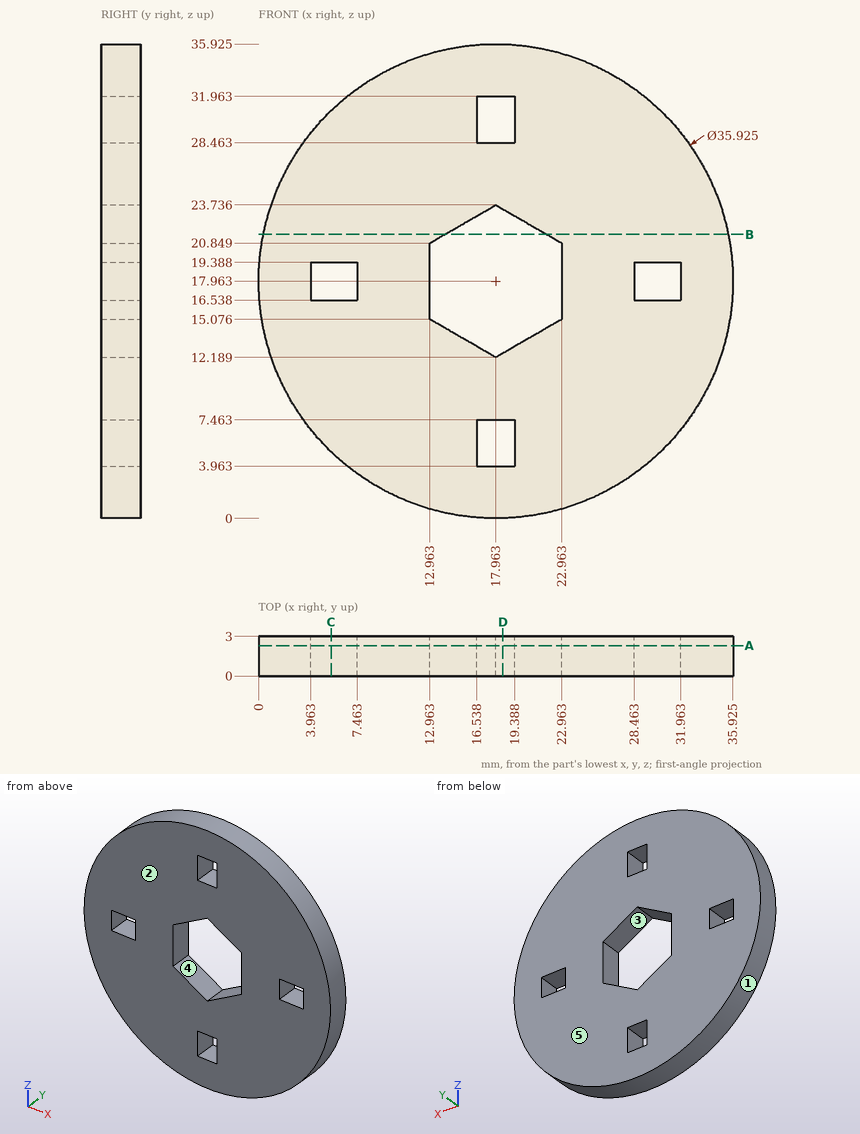
Answer from the drawing. Dimensions are ordinates in mm from the lowest x, y and z of the part. A direction names the side the tool comes from. Give positions to 0.01 mm unless a question says otherwise; leave off trailing zeros. Write each loop counter-clockwise with the first axis right and the second up, starting at its lowest first coordinate (ties: lowest second). Pieces come first, ordered by that corner, then holes. Notation, with made-up numbers: (18.25, 56) - (42.25, 56) arc R8 ccw to (42.25, 63) - close; hole circle Ø8 at (70.25, -13). An arc over 180 degrees is marked (long way). One line per item, written item: value. Start each with the question number.
1. For a pull along X with two mould halves and no side action, classify the marked faces 1, 2 and 3 as +X half, -X half, draft (parallel to the pull), parting line (faces both ways), or undercut.
2. Find section C-C (x = 5.5). Write down the section's boundary in (y, z).
3. Given pin 1 (0.9 mm diameter, centred on y = 1.5, z = 18.5, fed in from -X); pin 2 (1.5 mm diameter, centred on y = 2.5, z = 3.5, fed in from -X); pin 3 (0.9 mm diameter, centred on y = 1.5, z = 31, fed in from -X), each flat-ended and moving along its own axis, determine where each tip first touches the part or whether it passes through.
4. For the marked faces 4 and 5, determine the directions among +Z, -Z, +X, -X, +Y, -Y from which every point of the face is accessible in a straight line to the end or side of a thin tool.
5. Find section B-B (z = 21.5). Write down the section's boundary in (x, y).
6. Consider probe 1 along X at (y, z) = (2.4, 18) (1 decimal); probe 2 along Z at (x, y) = (17, 0.1) (1 decimal); probe 3 along X at (y, z) = (0.1, 16). Determine where each line is inside the solid, lowest interval first.
7. Find section D-D (x = 18.5). Write down the section's boundary in (y, z).
8. Find section A-A (y = 2.3). State how many separate pieces and enclosed holes the cut face has, then the cut area to 3 significant figures.
Geometry results:
1. face 1: parting line
1. face 2: draft
1. face 3: undercut
2. outline: (0, 5.03) - (3, 5.03) - (3, 16.54) - (0, 16.54) - close; (0, 19.39) - (3, 19.39) - (3, 30.9) - (0, 30.9) - close
3. pin 1: x = 0
3. pin 2: x = 6.36
3. pin 3: x = 5.15
4. face 4: +Y, -Y
4. face 5: +Z, -Z, +X, -X, +Y
5. outline: (0.35, 0) - (14.09, 0) - (14.09, 3) - (0.35, 3) - close; (21.84, 0) - (35.57, 0) - (35.57, 3) - (21.84, 3) - close
6. probe 1: 0 to 4, 7.5 to 13, 23 to 28.5, 32 to 35.9
6. probe 2: 0 to 4, 7.5 to 12.7, 23.2 to 28.5, 32 to 35.9
6. probe 3: 0.11 to 12.96, 22.96 to 35.82
7. outline: (0, 0.01) - (3, 0.01) - (3, 3.96) - (0, 3.96) - close; (0, 7.46) - (3, 7.46) - (3, 12.5) - (0, 12.5) - close; (0, 23.43) - (3, 23.43) - (3, 28.46) - (0, 28.46) - close; (0, 31.96) - (3, 31.96) - (3, 35.92) - (0, 35.92) - close
8. separate pieces: 1
8. enclosed holes: 5
8. area: 887 mm2
